from build123d import *

# Parameters (mm, degrees)
SKETCH1_R           = 2.5
BOSS_EXTRUDE1_DEPTH = 189.096108091
SCALE_2_SCALE       = 3
SCALE_3_SCALE       = 6
SCALE_5_SCALE       = 2
SCALE_6_SCALE       = 0.25
SCALE_7_SCALE       = 0.125
SCALE_8_SCALE       = 0.25
SCALE_9_SCALE       = 4
SCALE_10_SCALE      = 4
SCALE_11_SCALE      = 0.111111111


with BuildPart() as part:
    # Sketch1 → Boss-Extrude1 (new body)
    with BuildSketch(Plane.XY):
        with BuildLine():
            Line((2.839339828, 3.9), (5.5, 6.560660172))
            Line((5.5, 6.560660172), (5.5, 8.2))
            Line((5.5, 8.2), (3.1, 8.2))
            Line((3.1, 8.2), (3.1, 9.5))
            Line((3.1, 9.5), (3.6, 9.5))
            Line((3.6, 9.5), (3.6, 10))
            Line((3.6, 10), (8.5, 10))
            ThreePointArc((8.5, 10), (9.560660172, 9.560660172), (10, 8.5))
            Line((10, 8.5), (10, 3.6))
            Line((10, 3.6), (9.5, 3.6))
            Line((9.5, 3.6), (9.5, 3.1))
            Line((9.5, 3.1), (8.2, 3.1))
            Line((8.2, 3.1), (8.2, 5.5))
            Line((8.2, 5.5), (6.560660172, 5.5))
            Line((6.560660172, 5.5), (3.9, 2.839339828))
            Line((3.9, 2.839339828), (3.9, -2.839339828))
            Line((3.9, -2.839339828), (6.560660172, -5.5))
            Line((6.560660172, -5.5), (8.2, -5.5))
            Line((8.2, -5.5), (8.2, -3.1))
            Line((8.2, -3.1), (9.5, -3.1))
            Line((9.5, -3.1), (9.5, -3.6))
            Line((9.5, -3.6), (10, -3.6))
            Line((10, -3.6), (10, -8.5))
            ThreePointArc((10, -8.5), (9.560660172, -9.560660172), (8.5, -10))
            Line((8.5, -10), (3.6, -10))
            Line((3.6, -10), (3.6, -9.5))
            Line((3.6, -9.5), (3.1, -9.5))
            Line((3.1, -9.5), (3.1, -8.2))
            Line((3.1, -8.2), (5.5, -8.2))
            Line((5.5, -8.2), (5.5, -6.560660172))
            Line((5.5, -6.560660172), (2.839339828, -3.9))
            Line((2.839339828, -3.9), (-2.839339828, -3.9))
            Line((-2.839339828, -3.9), (-5.5, -6.560660172))
            Line((-5.5, -6.560660172), (-5.5, -8.2))
            Line((-5.5, -8.2), (-3.1, -8.2))
            Line((-3.1, -8.2), (-3.1, -9.5))
            Line((-3.1, -9.5), (-3.6, -9.5))
            Line((-3.6, -9.5), (-3.6, -10))
            Line((-3.6, -10), (-8.5, -10))
            ThreePointArc((-8.5, -10), (-9.560660172, -9.560660172), (-10, -8.5))
            Line((-10, -8.5), (-10, -3.6))
            Line((-10, -3.6), (-9.5, -3.6))
            Line((-9.5, -3.6), (-9.5, -3.1))
            Line((-9.5, -3.1), (-8.2, -3.1))
            Line((-8.2, -3.1), (-8.2, -5.5))
            Line((-8.2, -5.5), (-6.560660172, -5.5))
            Line((-6.560660172, -5.5), (-3.9, -2.839339828))
            Line((-3.9, -2.839339828), (-3.9, 2.839339828))
            Line((-3.9, 2.839339828), (-6.560660172, 5.5))
            Line((-6.560660172, 5.5), (-8.2, 5.5))
            Line((-8.2, 5.5), (-8.2, 3.1))
            Line((-8.2, 3.1), (-9.5, 3.1))
            Line((-9.5, 3.1), (-9.5, 3.6))
            Line((-9.5, 3.6), (-10, 3.6))
            Line((-10, 3.6), (-10, 8.5))
            ThreePointArc((-10, 8.5), (-9.560660172, 9.560660172), (-8.5, 10))
            Line((-8.5, 10), (-3.6, 10))
            Line((-3.6, 10), (-3.6, 9.5))
            Line((-3.6, 9.5), (-3.1, 9.5))
            Line((-3.1, 9.5), (-3.1, 8.2))
            Line((-3.1, 8.2), (-5.5, 8.2))
            Line((-5.5, 8.2), (-5.5, 6.560660172))
            Line((-5.5, 6.560660172), (-2.839339828, 3.9))
            Line((-2.839339828, 3.9), (2.839339828, 3.9))
        make_face()
        with Locations((0, 0.235847297)):
            Circle(SKETCH1_R, mode=Mode.SUBTRACT)
    extrude(amount=BOSS_EXTRUDE1_DEPTH)


with BuildPart() as part_1:
    # 缩放比例2: scaled about (0, -0.027095247, 94.548054046)
    add(part.part.scale(SCALE_2_SCALE).moved(Location((0, 0.054190494, -189.096108092))))


with BuildPart() as part_2:
    # 缩放比例3: scaled about (0, -0.027095247, 94.548054045)
    add(part_1.part.scale(SCALE_3_SCALE).moved(Location((0, 0.135476235, -472.740270225))))


with BuildPart() as part_3:
    # 缩放比例5: scaled about (0, -0.027095249, 94.548054043)
    add(part_2.part.scale(SCALE_5_SCALE).moved(Location((0, 0.027095249, -94.548054043))))


with BuildPart() as part_4:
    # 缩放比例6: scaled about (0, -0.027095249, 94.548054044)
    add(part_3.part.scale(SCALE_6_SCALE).moved(Location((0, -0.020321437, 70.911040533))))


with BuildPart() as part_5:
    # 缩放比例7: scaled about (0, -0.027095249, 94.548054044)
    add(part_4.part.scale(SCALE_7_SCALE).moved(Location((0, -0.023708343, 82.729547289))))


with BuildPart() as part_6:
    # 缩放比例8: scaled about (0, -0.027095249, 94.548054044)
    add(part_5.part.scale(SCALE_8_SCALE).moved(Location((0, -0.020321437, 70.911040533))))


with BuildPart() as part_7:
    # 缩放比例9: scaled about (0, -0.027095249, 94.548054044)
    add(part_6.part.scale(SCALE_9_SCALE).moved(Location((0, 0.081285747, -283.644162132))))


with BuildPart() as part_8:
    # 缩放比例10: scaled about (0, -0.027095249, 94.548054044)
    add(part_7.part.scale(SCALE_10_SCALE).moved(Location((0, 0.081285747, -283.644162132))))


with BuildPart() as part_9:
    # 缩放比例11: scaled about (0, -0.027095249, 94.548054044)
    add(part_8.part.scale(SCALE_11_SCALE).moved(Location((0, -0.024084666, 84.042714706))))


solid = part_9.part
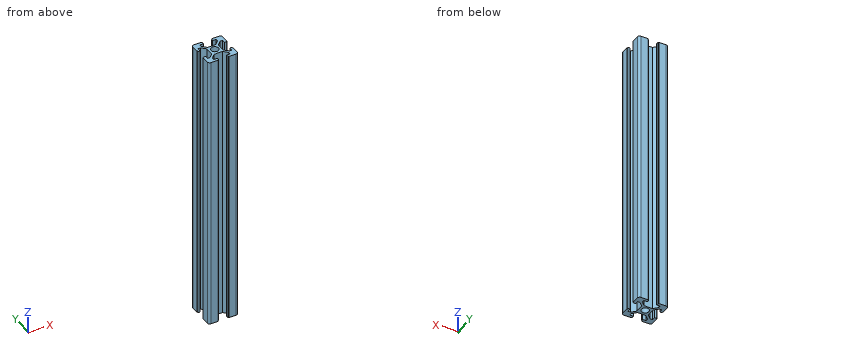
Here's how the part is built. I have some questions about the finished solid (model axes, mm). Round coordinates to 2 decimals unless told otherwise and drop trailing zeros. Loops run counter-clockwise (first coordinate to the right, second up) from the corner with the lowest first, then second, coordinate; pieces in that order, holes last.
1. For P1, Ø0.9, axis at y = 0, z = 105.5, coming from the -X side; P2, Ø2.5, axis at y = 0, z = 77, coming from the +X side; P3, Ø1.5, axis at x = -1, z = 82, coming from the -Y side, each with a flat end and sliding along its axis, tell me the tip position at first contact or that it passes through.
Answer list:
P1: stops at x = -1.95
P2: stops at x = 1.95
P3: stops at y = -4.76
2. If I drill on line 1 along X through (y, z) = (-4, 69); line 2 along Y through (x, z) = (0, 81); line 3 along Y through (x, z) = (4.25, 72), over which ranges is the centre line in solid material (lowest first)?
Answer list:
line 1: x = -5 to -2.75, 2.75 to 5
line 2: y = -1.96 to -1.15, 1.35 to 1.94
line 3: y = -5.01 to -1.56, 1.54 to 4.99
3. If we section it at A-A on x = 0: Write out the boundary of the cut face in (y, z).
Answer list:
outline: (-1.96, 47.27) - (-1.15, 47.27) - (-1.15, 141.82) - (-1.96, 141.82) - close; (1.35, 47.27) - (1.94, 47.27) - (1.94, 141.82) - (1.35, 141.82) - close
